from build123d import *

# Parameters (mm, degrees)
SZKIC1_W                    = 42
SZKIC1_H                    = 42
DODANIE_WYCI_GNI_CIE1_DEPTH = 33
SFAZOWANIE1_SIZE            = 4
SZKIC2_R                    = 11
DODANIE_WYCI_GNI_CIE2_DEPTH = 1.3
SZKIC3_R                    = 2.5
DODANIE_WYCI_GNI_CIE3_DEPTH = 21.75
SZKIC4_R                    = 1.5
WYTNIJ_WYCI_GNI_CIE1_DEPTH  = 34


with BuildPart() as part:
    # Szkic1 → Dodanie-wyciągnięcie1 (new body)
    with BuildSketch(Plane.XY):
        Rectangle(SZKIC1_W, SZKIC1_H)
    extrude(amount=DODANIE_WYCI_GNI_CIE1_DEPTH)

    # Sfazowanie1
    sfazowanie1_edges = [part.edges().sort_by_distance(p)[0] for p in [
        (21, -21, 16.5),
        (-21, -21, 16.5),
        (-21, 21, 16.5),
        (21, 21, 16.5),
    ]]
    chamfer(sfazowanie1_edges, length=SFAZOWANIE1_SIZE)

    # Szkic2 → Dodanie-wyciągnięcie2 (add)
    with BuildSketch(Plane(origin=(0, 0, 0), x_dir=(-1, 0, 0), z_dir=(0, 0, -1))):
        Circle(SZKIC2_R)
    extrude(amount=DODANIE_WYCI_GNI_CIE2_DEPTH)

    # Szkic3 → Dodanie-wyciągnięcie3 (add)
    with BuildSketch(Plane(origin=(0, 0, -1.3), x_dir=(-1, 0, 0), z_dir=(0, 0, -1))):
        Circle(SZKIC3_R)
    extrude(amount=DODANIE_WYCI_GNI_CIE3_DEPTH)

    # Szkic4 → Wytnij-wyciągnięcie1 (cut, through all)
    with BuildSketch(Plane(origin=(0, 0, 0), x_dir=(-1, 0, 0), z_dir=(0, 0, -1))):
        with Locations((15.5, 15.5)):
            Circle(SZKIC4_R)
        with Locations((-15.5, 15.5)):
            Circle(SZKIC4_R)
        with Locations((-15.5, -15.5)):
            Circle(SZKIC4_R)
        with Locations((15.5, -15.5)):
            Circle(SZKIC4_R)
    extrude(amount=-WYTNIJ_WYCI_GNI_CIE1_DEPTH, mode=Mode.SUBTRACT)


solid = part.part
The listing builds one solid part. Answer for the finished solid, in the listing's coordinates (mm). A direction names the side the tool comes from. Coordinates: 2 decimals unless noted, no trailing zeros. Loops run counter-clockwise (first coordinate to the right, second up) from the corner with the lowest first, then second, coordinate; pieces in that order, holes last. Notation, with made-up numbers: M -23,-20 L 4,-20 A8 cw 4,-6 Z; hole C 10,3 d6. An arc over 180 degrees is marked long. Answer in a Markdown table with one row per item.
1) Which of the six approach directions +Z, -Z, +X, -X, +Y, -Y give full straight-line access (tool end or side, diameter ignored) to faces 4 (the cylindrical face through (-14, -15.43, 16.27)), 5 (the cylindrical face through (2.38, -10.74, -0.64))?
Answers below:
| item | result |
|---|---|
| face 4 | +Z, -Z |
| face 5 | -Z |
2) Determine the mould class of faces 1 (the flat face through (0, -21, 16)), 2 (the cylindrical face through (17, 15.57, 16.27)), 3 (the flat face through (19, 19, 16)) for opening direction Y: released by +Y, released by -Y, zero draft, split by the parting line, or undercut.
Answers below:
| item | result |
|---|---|
| face 1 | released by -Y |
| face 2 | undercut |
| face 3 | released by +Y |
3) Find the intervals of material crossed by probe 1 along Y at (x, z) = (-15.5, 11); probe 2 along X at (y, z) = (15, 25); probe 3 along Z at (x, y) = (17, 12), in increasing order.
Answers below:
| item | result |
|---|---|
| probe 1 | -21 to -17, -14 to 14, 17 to 21 |
| probe 2 | -21 to -16.91, -14.09 to 14.09, 16.91 to 21 |
| probe 3 | 0 to 33 |
4) Find section A-A (y = -15.5). Determine the outline of the cut face in (x, z).
Answers below:
| item | result |
|---|---|
| outline | M -21,0 L -17,0 L -17,33 L -21,33 Z; M -14,0 L 14,0 L 14,33 L -14,33 Z; M 17,0 L 21,0 L 21,33 L 17,33 Z |
5) Find section D-D (x = 0). Determine the outline of the cut face in (y, z).
Answers below:
| item | result |
|---|---|
| outline | M -21,0 L -11,0 L -11,-1.3 L -2.5,-1.3 L -2.5,-23.05 L 2.5,-23.05 L 2.5,-1.3 L 11,-1.3 L 11,0 L 21,0 L 21,33 L -21,33 Z |
6) Find section B-B (z = 9). Determine the outline of the cut face in (x, y), then the cut area to 3 significant figures.
Answers below:
| item | result |
|---|---|
| outline | M -21,-17 L -17,-21 L 17,-21 L 21,-17 L 21,17 L 17,21 L -17,21 L -21,17 Z; hole C -15.5,-15.5 d3; hole C -15.5,15.5 d3; hole C 15.5,-15.5 d3; hole C 15.5,15.5 d3 |
| area | 1,700 mm^2 |
7) Given pin 1 (3 mm diameter, centred on x = 0, z = -6.5, fed in from -Y); pin 2 (12.5 mm diameter, centred on x = 5.5, y = -7.5, fed in from -Z); pin 3 (1.8 mm diameter, centred on x = 15.5, y = 15.5, fed in from +Z); pin 4 (5 mm diameter, centred on x = 6.5, z = -3, fed in from +Y), each flat-ended and moving along its own axis, determine where each tip first touches the part or whether it passes through.
Answers below:
| item | result |
|---|---|
| pin 1 | y = -2.5 |
| pin 2 | z = -1.3 |
| pin 3 | through |
| pin 4 | y = 9.96 |
